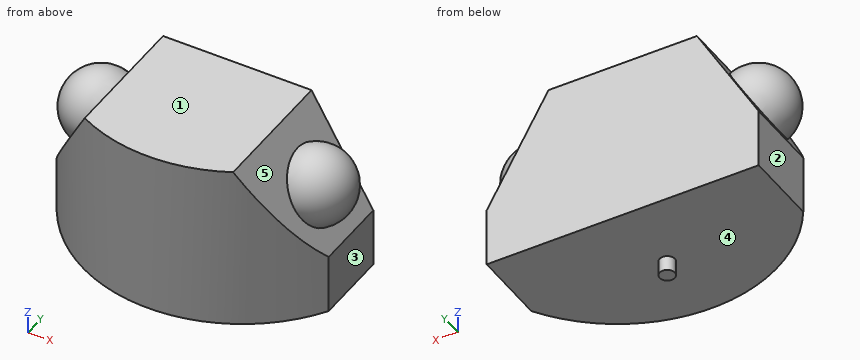
```python
from build123d import *

# Parameters (mm, degrees)
SKETCH1_W                = 180
SKETCH1_H                = 110
BOSS_EXTRUDE1_DEPTH      = 50
BOSS_EXTRUDE2_DEPTH      = 110
CUT_EXTRUDE1_DEPTH       = 146.344418537
BOSS_EXTRUDE5_DEPTH      = 10
BOSS_EXTRUDE5_DEPTH_BACK = 10
SKETCH5_R                = 5


with BuildPart() as part:
    # Sketch1 → Boss-Extrude1 (new body)
    with BuildSketch(Plane(origin=(0, 0, 0), x_dir=(1, 0, 0), z_dir=(0, 1, 0))):
        Rectangle(SKETCH1_W, SKETCH1_H)
    extrude(amount=BOSS_EXTRUDE1_DEPTH)

    # Sketch2 → Boss-Extrude2 (add)
    with BuildSketch(Plane(origin=(-35, 0, -55), x_dir=(1, 0, 0), z_dir=(0, 0, 1))):
        with BuildLine():
            Line((-55, 0), (125, 0))
            ThreePointArc((125, 0), (35, -50), (-55, 0))
        make_face()
    extrude(amount=BOSS_EXTRUDE2_DEPTH)

    # Sketch3 → Cut-Extrude1 (cut, through all)
    with BuildSketch(Plane(origin=(0, 50, 0), x_dir=(1, 0, 0), z_dir=(0, 1, 0))):
        Polygon((-49.118803686, -55), (-90, 15.808309091), (-90, -55), align=None)
    cut_extrude1 = extrude(amount=-CUT_EXTRUDE1_DEPTH, mode=Mode.SUBTRACT)

    # Mirror1: Cut-Extrude1 across plane
    add(cut_extrude1.mirror(Plane(origin=(0, 0, 0), x_dir=(0, 0, 1), z_dir=(1, 0, 0))), mode=Mode.SUBTRACT)

    # Sketch5 → Boss-Extrude5 (add, two sides: drawn at the far end of the back side and taken through both)
    with BuildSketch(Plane(origin=(0, 0, -55), x_dir=(-1, 0, 0), z_dir=(0, 0, -1)).offset(-BOSS_EXTRUDE5_DEPTH_BACK)):
        Circle(SKETCH5_R)
    extrude(amount=BOSS_EXTRUDE5_DEPTH + BOSS_EXTRUDE5_DEPTH_BACK)

    # Sketch4 → Revolve1 (revolve)
    with BuildSketch(Plane(origin=(-60.654801368, 0, 35.019065898), x_dir=(0.49999999999999495, 0, 0.8660254037844417), z_dir=(-0.8660254037844417, 0, 0.49999999999999495))):
        with BuildLine():
            ThreePointArc((-20.965161058, 42.942576489), (4.034838942, 17.942576489), (-20.965161058, -7.057423511))
            Line((-20.965161058, -7.057423511), (-20.965161058, 42.942576489))
        make_face()
    revolve1 = revolve(axis=Axis((-71.137381897, 42.942576489, 16.862703827), (0, -1, 0)))

    # Mirror2: Revolve1 across plane
    add(revolve1.mirror(Plane(origin=(0, 0, 0), x_dir=(0, 0, 1), z_dir=(1, 0, 0))))


solid = part.part
```
Source: CAD feature listing. Evaluate the final solid. Frame: model axes, mm. Face numbers are marked on the shaded views. A direction names the side the tool comes from. Round coordinates to 2 decimals unless told otherwise and drop trailing zeros. Loops run counter-clockwise (first coordinate to the right, second up) from the corner with the lowest first, then second, coordinate; pieces in that order, holes last. Notation, with made-up numbers: M 49.25,42 L 102.25,42 A31 ccw 102.25,71 Z; hole C 29.5,-34 d7. An arc over 180 degrees is marked long. Use a Markdown table: item, result. Add a question column.
1. Reachability of the marked faces 1 and 2 from +Z, -Z, +X, -X, +Y, -Y: full face, straight path, thin tool, end or side. Return the list, or none.
2. Section query B-B on y = -18. Return the cut outline in (x, z), then the cut area to 3 significant figures.
3. Section query C-C on z = -21. Return the cut outline in (x, y), then the cut area to 3 significant figures.
4. Mould query, pull axis Z, two halves, no side actions, for the marked faces 3, 4 and 5. Classes: pulls with the +Z half, pulls with the -Z half, needs draft (parallel to the pull), parting line crosses it, or undercut.
5. Section query A-A on x = 0. Return the cut outline in (y, z).
6. Contact query for flat-ended pins moving along their axis: P1, Ø1, axis at y = 7.5, z = -27, coming from the -X side; P2, Ø4, axis at y = 6, z = -5, coming from the -X side; P3, Ø6, axis at x = -72, z = -40.5, coming from the -Y side. Output: stop coordinate, or through.
7. Section query D-D on y = 27. Return the cut outline in (x, z).
8. Line query: line 1 (Z direction, x = 10, y = 35.5); line 2 (X direction, y = 27, z = -16.5); line 3 (Z direction, x = -52, y = 20). Output: solid intervals per line, ascending.
Reported:
| question | item | result |
|---|---|---|
| 1 | face 1 | +Z, +X, -X, +Y, -Y |
| 1 | face 2 | -Z, -X, +Y, -Y |
| 2 | outline | M -75.89,-55 L 75.89,-55 L 75.89,8.62 L 49.12,55 L -49.12,55 L -75.89,8.62 Z |
| 2 | area | 15,500 mm² |
| 3 | outline | M -90,0 A106 ccw 90,0 L 90,50 L -90,50 Z |
| 3 | area | 15,400 mm² |
| 4 | face 3 | needs draft |
| 4 | face 4 | pulls with the -Z half |
| 4 | face 5 | undercut |
| 5 | outline | M -50,-55 L -5,-55 L -5,-65 L 5,-65 L 5,-55 L 50,-55 L 50,55 L -50,55 Z |
| 6 | P1 | stops at x = -90 |
| 6 | P2 | stops at x = -84.91 |
| 6 | P3 | stops at y = -24.47 |
| 7 | outline | M -90,-55 L 90,-55 L 90,-15.81 L 82.79,-3.32 A23.3 ccw 59.49,37.04 L 49.12,55 L -49.12,55 L -59.49,37.04 A23.3 ccw -82.79,-3.32 L -90,-15.81 Z |
| 8 | line 1 | z = -55 to 55 |
| 8 | line 2 | x = -90 to 90 |
| 8 | line 3 | z = -55 to 50.01 |
